CAD build for the part. Positions are in the model's coordinates, mm. A direction names the side the tool comes from. Round coordinates to 2 decimals unless told otherwise and drop trailing zeros. Write each loop counter-clockwise with the first axis right and the second up, starting at its lowest first coordinate (ties: lowest second). Pieces come first, ordered by that corner, then holes. Notation, with made-up numbers: (50.5, 34) - (103.5, 34) arc R26 cw to (103.5, 71) - close; hole circle Ø11 at (13, 55.5). An arc over 180 degrees is marked (long way). Put each result on its own line as item: value. Start each with the question number.
Item 1: Drill centre lines: line 1 (Y direction, x = 0, z = 9.25); line 2 (Y direction, x = 4.25, z = 10.75); line 3 (X direction, y = -16, z = 6.75). Where is each one in solid material? Low to high. Write a range as from..to.
Item 2: 3-axis set-ups, long thin cutter, end or side, ignore diameter. For faces 1 (the flat face through (0, -35, 0)), 2 (the flat face through (12, -2.506, 6)), 3 (the flat face through (0, 6.494, 6)), 4 (the flat face through (-10, 4, 6)), 5 (the flat face through (-10, -20, 6)): which of +Z, -Z, +X, -X, +Y, -Y reach the whole face in a straight line?
Item 3: Cut at A-A (x = 0). Give the cut face in (y, z), and give its area (3 significant figures).
Item 4: Cut at D-D (x = -5.5). Give the cut face in (y, z), and give its area (3 significant figures).
Item 5: Cut at B-B (z = 6). Give the cut face in (x, y) (3 decimals).
Item 6: Cut at C-C (z = 9). Give the cut face in (x, y) (3 decimals).
Item 7: Pin check, flat tips, straight feed: pin 1 Ø5.5 at (x, z) = (12, 7.5) entering from +Y; pin 2 Ø3.5 at (x, z) = (-3, 8.5) entering from -Y; pin 3 Ø6 at (y, z) = (-53, 9) entering from -X; pin 4 Ø4 at (y, z) = (1.49, 6) entering from +X. Stop position of each tip, or through.
Item 8: Mould opens along X. For faces 6 (the flat face through (10, -20, 6)), 7 (the cylindrical face through (-2.1, -56.9, 5.9)), 8 (the flat face through (0, -35, 12)), 9 (the flat face through (10, 4, 6)) say: released by +X, released by -X, zero draft, split by the parting line, or undercut.
```python
from build123d import *

# Parameters (mm, degrees)
SKETCH1_R           = 9.625
SKETCH1_W           = 20
SKETCH1_H           = 25
BOSS_EXTRUDE1_DEPTH = 12
SKETCH2_R           = 2.25
CUT_EXTRUDE1_DEPTH  = 69.381198132


with BuildPart() as part:
    # Sketch1 → Boss-Extrude1 (new body)
    with BuildSketch(Plane.XY):
        with BuildLine():
            Line((-10, -2.505905785), (-10, 6.494094215))
            Line((-10, 6.494094215), (10, 6.494094215))
            Line((10, 6.494094215), (10, -2.505905785))
            Line((10, -2.505905785), (15, -2.505905785))
            Line((15, -2.505905785), (15, -47.505905785))
            ThreePointArc((15, -47.505905785), (0, -62.505905785), (-15, -47.505905785))
            Line((-15, -47.505905785), (-15, -2.505905785))
            Line((-15, -2.505905785), (-10, -2.505905785))
        make_face()
        with Locations((0, -47.505905785)):
            Circle(SKETCH1_R, mode=Mode.SUBTRACT)
        with Locations((0, -20.005905785)):
            Rectangle(SKETCH1_W, SKETCH1_H, mode=Mode.SUBTRACT)
    extrude(amount=BOSS_EXTRUDE1_DEPTH)

    # Sketch2 → Cut-Extrude1 (cut, through all)
    with BuildSketch(Plane(origin=(10, 0, 0), x_dir=(0, 0, -1), z_dir=(1, 0, 0))):
        with Locations(Location((-6, 1.494094215, 0), (0, 0, 90))):
            Circle(SKETCH2_R)
    extrude(amount=-CUT_EXTRUDE1_DEPTH, mode=Mode.SUBTRACT)


solid = part.part
```
Output values:
1. line 1: -62.51..-57.13, -37.88..-32.51, -7.51..6.49
1. line 2: -61.89..-56.14, -38.87..-32.51, -7.51..6.49
1. line 3: -15..-10, 10..15
2. face 1: -Z, +X, -X, +Y, -Y
2. face 2: +Z, -Z, +X, +Y
2. face 3: +Z, -Z, +X, -X, +Y
2. face 4: +Z, -Z, -X, +Y
2. face 5: +Z, -Z
3. outline: (-62.51, 0) - (-57.13, 0) - (-57.13, 12) - (-62.51, 12) - close; (-37.88, 0) - (-32.51, 0) - (-32.51, 12) - (-37.88, 12) - close; (-7.51, 0) - (6.49, 0) - (6.49, 12) - (-7.51, 12) - close; hole circle Ø4.5 at (1.49, 6)
3. area: 281 mm2
4. outline: (-61.46, 0) - (-55.4, 0) - (-55.4, 12) - (-61.46, 12) - close; (-39.61, 0) - (-32.51, 0) - (-32.51, 12) - (-39.61, 12) - close; (-7.51, 0) - (6.49, 0) - (6.49, 12) - (-7.51, 12) - close; hole circle Ø4.5 at (1.49, 6)
4. area: 310 mm2
5. outline: (-15, -47.506) arc R15 ccw to (15, -47.506) - (15, -2.506) - (10, -2.506) - (10, -0.756) - (-10, -0.756) - (-10, -2.506) - (-15, -2.506) - close; (-10, 3.744) - (10, 3.744) - (10, 6.494) - (-10, 6.494) - close; hole (-10, -32.506) - (10, -32.506) - (10, -7.506) - (-10, -7.506) - close; hole circle Ø19.25 at (0, -47.506)
6. outline: (-15, -47.506) arc R15 ccw to (15, -47.506) - (15, -2.506) - (10, -2.506) - (10, 6.494) - (-10, 6.494) - (-10, -2.506) - (-15, -2.506) - close; hole (-10, -32.506) - (10, -32.506) - (10, -7.506) - (-10, -7.506) - close; hole circle Ø19.25 at (0, -47.506)
7. pin 1: y = 6.49
7. pin 2: y = -62.45
7. pin 3: x = -14.79
7. pin 4: through
8. face 6: undercut
8. face 7: undercut
8. face 8: zero draft
8. face 9: released by +X
